```python
from build123d import *

# Parameters (mm, degrees)
KEYWAY_DEPTH       = 2.38125
SKETCH3_OUTSIDE_W  = 58.716
SKETCH3_OUTSIDE_H  = 58.716
CUT_EXTRUDE2_DEPTH = 12.7


with BuildPart() as part:
    # Sketch1 → Base (revolve)
    with BuildSketch(Plane.XY, mode=Mode.PRIVATE) as base_sk:
        Polygon((0, 0), (0, 6.35), (12.7, 6.35), (12.7, 7.9375), (26.9875, 7.9375), (26.9875, 6.35), (28.575, 6.35), (28.575, 7.9375), (146.05, 7.9375), (146.05, 12.7), (152.4, 12.7), (152.4, 0), align=None)
    revolve(base_sk.sketch.rotate(Axis((0, 0, 0), (-1, 0, 0)), 90), axis=Axis((0, 0, 0), (-1, 0, 0)))

    # Sketch2 → Keyway (cut, symmetric)
    with BuildSketch(Plane.XY):
        with BuildLine():
            Line((69.85, 14.2875), (69.85, 8.7249))
            ThreePointArc((69.85, 8.7249), (70.77993597, 6.47983597), (73.025, 5.5499))
            Line((73.025, 5.5499), (101.6, 5.5499))
            ThreePointArc((101.6, 5.5499), (103.84506403, 6.47983597), (104.775, 8.7249))
            Line((104.775, 8.7249), (104.775, 14.2875))
            Line((104.775, 14.2875), (69.85, 14.2875))
        make_face()
    extrude(amount=KEYWAY_DEPTH, both=True, mode=Mode.SUBTRACT)

    # Sketch3 outside → Cut-Extrude2 (cut)
    with BuildSketch(Plane.ZY):
        Rectangle(SKETCH3_OUTSIDE_W, SKETCH3_OUTSIDE_H)
        Polygon((3.175, 5.499261314), (-3.175, 5.499261314), (-6.35, 0), (-3.175, -5.499261314), (3.175, -5.499261314), (6.35, 0), align=None, mode=Mode.SUBTRACT)
    extrude(amount=-CUT_EXTRUDE2_DEPTH, mode=Mode.SUBTRACT)


solid = part.part
```
The model under review builds one solid part; all positions refer to its coordinate system, in mm. A direction names the side the tool comes from. Coordinates: 2 decimals unless noted, no trailing zeros. Write each loop counter-clockwise with the first axis right and the second up, starting at its lowest first coordinate (ties: lowest second). Pieces come first, ordered by that corner, then holes. Notation, with made-up numbers: (78, -1.75) -> (126, -1.75) arc R36 cw to (126, 37.25) -> close; hole circle Ø4 at (-28, 75.5). An arc over 180 degrees is marked (long way). One line per item, written item: value. Start each with the question number.
Q1. To check wall thickness, follow probe 1 along X at (y, z) = (9.25, 5.75); probe 2 along Y at (x, z) = (36.5, 0); probe 3 along Y at (x, z) = (8.5, 1.5). State the ranges of each line that lie inside material, in increasing order.
Q2. For faces 1 (the face through (26.988, -7, 0)), 2 (the face through (6.261, 2.711, 4.785)), 3 (the face through (146.05, 8.3, -0.2)), list the 3-axis set-ups (+Z, -Z, +X, -X, +Y, -Y) from which the entire face can be reached by the end or side of a thin tool; tool diameter is ignored.
Q3. Add section B-B, the plane x = 98.5. Give the boundary of the cut face in (y, z) (1 decimal).
Q4. Add section D-D, the plane x = 122. Give the boundary of the cut face in (y, z) (1 decimal).
Q5. Clearance check with flat-ended pins moving along their axes: P1, Ø1.9, axis at x = 7.5, z = 1.5, coming from the -Y side; P2, Ø1.5, axis at x = 45, z = 3.5, coming from the -Y side; P3, Ø7, axis at x = 6.5, z = 1, coming from the +Y side. State where each tip first meets the part, or that it passes through.
Q6. The part is to be moulded in two halves that separate along X. For faces 4 (the face through (27.79, 3.86, 5.04)), 5 (the face through (0, 0, 0)), 6 (the face through (6.26, 2.79, -4.74)), say which applies: +X half, -X half, draft (parallel to the pull), parting line (faces both ways), or undercut.
Response:
1. probe 1: 146.05 to 152.4
1. probe 2: -7.94 to 7.94
1. probe 3: -5.5 to 5.5
2. face 1: none
2. face 2: +Z, -X, +Y
2. face 3: -X
3. outline: (5.5, -2.4) -> (5.5, 2.4) -> (7.6, 2.4) arc R7.9 ccw (long way) to (7.6, -2.4) -> close
4. outline: circle Ø15.9 at (0, 0)
5. P1: y = -5.5
5. P2: y = -7.45
5. P3: y = 5.5
6. face 4: undercut
6. face 5: -X half
6. face 6: draft
